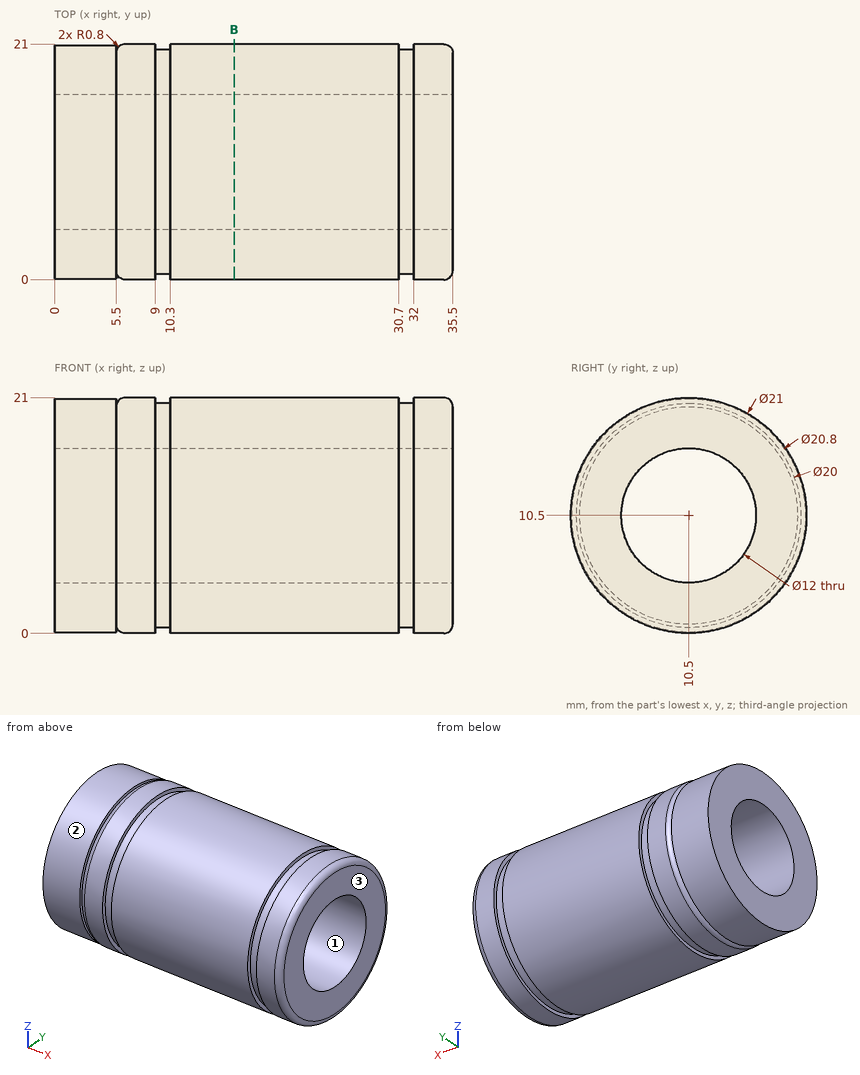
Geometry check sheet. Reference: drawing and pictorial views, mm from the part's lowest x, y, z. Give positions to 0.01 mm unless a question says otherwise; leave off trailing zeros. Write each loop counter-clockwise with the first axis right and the second up, starting at its lowest first coordinate (ties: lowest second). Pieces come first, ordered by that corner, then holes. Notation, with made-up numbers: (20.25, 68.5) - (51.25, 68.5) arc R10 ccw to (51.25, 82.5) - close; hole circle Ø5 at (43, -33.75). An arc over 180 degrees is marked (long way). Put each result on its own line as item: value.
Q1. Scan lines: probe 1 along Y at (x, z) = (18.5, 10.5); probe 2 along Y at (x, z) = (12, 6); probe 3 along Z at (x, y) = (14, 14). Record each from-to range of solid material in increasing order. Write a range as from..to.
Result:
probe 1: 0..4.5, 16.5..21
probe 2: 1.01..6.53, 14.47..19.99
probe 3: 0.6..5.63, 15.37..20.4
Q2. Mould release check, pull along Z, two halves, no side actions. Record for the marked faces 1, 2 and 3: released by +Z, released by -Z, zero draft, split by the parting line, or undercut.
Result:
face 1: undercut
face 2: split by the parting line
face 3: zero draft
Q3. Section check B-B on x = 16. Record the cut outline in (y, z), and give its area (3 significant figures).
Result:
outline: circle Ø21 at (10.5, 10.5); hole circle Ø12 at (10.5, 10.5)
area: 233 mm2
Q4. Depth check by flat-ended pin: P1, Ø8, axis at x = 23.5, y = 6, coming from the +Z side; P2, Ø2, axis at y = 16, z = 2.5, coming from the -X side; P3, Ø5, axis at x = 25.5, z = 14, coming from the -Y side; P4, Ø10, axis at x = 13, z = 18, coming from the +Y side. Enter the tip coordinate at first touch or a pass-through.
Result:
P1: z = 20.99
P2: x = 0
P3: y = 0.05
P4: y = 20.7
